Geometry: final body of the model. Coordinates: model frame, mm. Coordinates: 2 decimals unless noted, no trailing zeros. Write each loop counter-clockwise with the first axis right and the second up, starting at its lowest first coordinate (ties: lowest second). Pieces come first, ordered by that corner, then holes. Notation, with made-up numbers: (9, -35.75) -> (55, -35.75) arc R32 cw to (55, -5.75) -> close; hole circle Ø2 at (24.25, -12). An arc over 180 degrees is marked (long way). Answer as a JSON object with one key per item and string values. Group by question number.
Autodesk Inventor part; units mm, degrees
ref_plane "YZ Plane" through (0, 0, 0) normal (1, 0, 0) x (0, 1, 0)
ref_plane "XZ Plane" through (0, 0, 0) normal (0, 1, 0) x (-1, 0, 0)
ref_plane "XY Plane" through (0, 0, 0) normal (0, 0, 1) x (1, 0, 0)
sketch "Szkic1" plane through (0, 0, 0) normal (1, 0, 0) x (0, 1, 0)
  line L0 (-32.5, 103) -> (32.5, 103)
  line L1 (38.5, 97) -> (38.5, -97)
  line L2 (32.5, -103) -> (-32.5, -103)
  line L3 (-38.5, -97) -> (-38.5, 97)
  line L4 (-38.5, 103) -> (38.5, -103) construction
  arc A0 (32.5, -103) -> (38.5, -97) centre (32.5, -97) ccw
  arc A1 (-32.5, 103) -> (-38.5, 97) centre (-32.5, 97) ccw
  arc A2 (-38.5, -97) -> (-32.5, -103) centre (-32.5, -97) ccw
  arc A3 (38.5, 97) -> (32.5, 103) centre (32.5, 97) ccw
  point P0 (0, 0)
  dimension "d3" = 6
extrude "Płyta1" add sketch "Szkic1" along normal blind 3
sketch "Szkic2" plane through (3, 0, 0) normal (1, 0, 0) x (0, 0, -1)
  line L0 (-97, 38.5) -> (97, 38.5)
  line L1 (-103, -32.5) -> (-103, 32.5)
  line L2 (103, 32.5) -> (103, -32.5)
  line L3 (97, -38.5) -> (-97, -38.5)
  point P0 (0, 0)
  point P1 (-53, 25.5)
  point P2 (53, 25.5)
  point P3 (53, -25.5)
  point P4 (-53, -25.5)
  dimension "d5" = 13
  dimension "d6" = 50
  dimension "d7" = 50
  dimension "d8" = 13
  dimension "d9" = 50
  dimension "d10" = 13
  dimension "d11" = 13
  dimension "d12" = 50
hole "Otwór1" at (3, -25.5, 53) at (3, 25.5, 53) at (3, 25.5, -53) at (3, -25.5, -53) direction (-1, 0, 0) diameter 5.5 depth 3 tip angle 118
equation "\"d18\" = Grubość"
equation "\"d4\" = Grubość"
equation "\"PromieńGięcia\" = Grubość"
equation "\"SzerokośćGięciaPodcięcia\" = Grubość"
equation "\"GłębokośćGięciaPodcięcia\" = 0.5 * Grubość"
equation "\"RozmiarPodcięciaNarożnika\" = 4 * Grubość"
equation "\"MinimalnaPozostałość\" = 2 * Grubość"
equation "\"PromieńPrzejścia\" = PromieńGięcia"
equation "\"Rozmiar_promienia_Jacobiego\" = PromieńGięcia"
equation "\"Wielk_odstępu\" = Grubość"
properties part number "ZaslepkaObudowa" material "Aluminum 6061"
Item 1: Contact query for flat-ended pins moving along their axis: pin 1 (7 mm diameter, centred on y = 25.5, z = -53, fed in from -X); pin 2 (3.5 mm diameter, centred on y = -25.5, z = 53, fed in from +X). Output: stop coordinate, or through.
Item 2: Section A-A on y = -25.5. Output: boundary loops of the cut face in (x, z).
Item 3: Mould query, pull axis Y, two halves, no side actions, for faces 1 (the cylindrical face through (1.479, 36.789, -101.196)), 2 (the flat face through (0, -1, 1)), 3 (the cylindrical face through (1.479, -25.621, 55.747)). Classes: +Y half, -Y half, draft (parallel to the pull), parting line (faces both ways), or undercut.
Item 4: Ray query, L1, parallel to Y at x = 1.95, z = -53; L2, parallel to Z at x = 1.8, y = -25.5. Return the intervals inside material, ascending. Write a range as [from, to].
Item 5: Section B-B on z = 53. Output: boundary loops of the cut face in (x, y), then the cut area to 3 significant figures.
Answer sheet:
{
 "1": {"pin 1": "stops at x = 0", "pin 2": "passes through"},
 "2": {"outline": "(0, -103) -> (3, -103) -> (3, -55.75) -> (0, -55.75) -> close; (0, -50.25) -> (3, -50.25) -> (3, 50.25) -> (0, 50.25) -> close; (0, 55.75) -> (3, 55.75) -> (3, 103) -> (0, 103) -> close"},
 "3": {"face 1": "+Y half", "face 2": "draft", "face 3": "undercut"},
 "4": {"L1": "y = [-38.5, -28.25], [-22.75, 22.75], [28.25, 38.5]", "L2": "z = [-103, -55.75], [-50.25, 50.25], [55.75, 103]"},
 "5": {"outline": "(0, -38.5) -> (3, -38.5) -> (3, -28.25) -> (0, -28.25) -> close; (0, -22.75) -> (3, -22.75) -> (3, 22.75) -> (0, 22.75) -> close; (0, 28.25) -> (3, 28.25) -> (3, 38.5) -> (0, 38.5) -> close", "area": "198 mm^2"}
}
